from build123d import *

# Parameters (mm, degrees)
SKETCH1_W           = 56.388
SKETCH1_H           = 45.72
BOSS_EXTRUDE1_DEPTH = 2.54
SKETCH2_W           = 2.7432
SKETCH2_H           = 19.05
BOSS_EXTRUDE2_DEPTH = 2.54
SKETCH3_W           = 19.05
SKETCH3_H           = 2.7432
CUT_EXTRUDE1_DEPTH  = 3.54
SKETCH4_R           = 3.937
CUT_EXTRUDE2_DEPTH  = 3.54


with BuildPart() as part:
    # Sketch1 → Boss-Extrude1 (new body)
    with BuildSketch(Plane(origin=(0, 0, 0), x_dir=(0, 0, -1), z_dir=(1, 0, 0))):
        Rectangle(SKETCH1_W, SKETCH1_H)
    extrude(amount=BOSS_EXTRUDE1_DEPTH)

    # Sketch2 → Boss-Extrude2 (add)
    with BuildSketch(Plane(origin=(2.54, 0, 0), x_dir=(0, 0, -1), z_dir=(1, 0, 0))):
        with Locations((-29.5656, 0)):
            Rectangle(SKETCH2_W, SKETCH2_H)
        with Locations((29.5656, 0)):
            Rectangle(SKETCH2_W, SKETCH2_H)
    extrude(amount=-BOSS_EXTRUDE2_DEPTH)

    # Sketch3 → Cut-Extrude1 (cut, through all)
    with BuildSketch(Plane(origin=(2.54, 0, 0), x_dir=(0, 0, -1), z_dir=(1, 0, 0))):
        with Locations((0, 21.4884)):
            Rectangle(SKETCH3_W, SKETCH3_H)
        with Locations((0, -14.7066)):
            Rectangle(SKETCH3_W, SKETCH3_H)
    extrude(amount=-CUT_EXTRUDE1_DEPTH, mode=Mode.SUBTRACT)

    # Sketch4 → Cut-Extrude2 (cut, through all)
    with BuildSketch(Plane(origin=(2.54, 0, 0), x_dir=(0, 0, -1), z_dir=(1, 0, 0))):
        with Locations((11.8872, 10.16)):
            Circle(SKETCH4_R)
    extrude(amount=-CUT_EXTRUDE2_DEPTH, mode=Mode.SUBTRACT)


solid = part.part
Check sheet for the modelled part. Datum: model origin and axes. Units: mm. A direction names the side the tool comes from. Round coordinates to 2 decimals unless told otherwise and drop trailing zeros. Order: outer loops, then holes, each group sorted by start corner. A loop starts at its lowest first (then second) coordinate and runs counter-clockwise, first axis right, second up.
(1) Go/stop test with flat-tipped pins: P1, Ø1.3, axis at x = 2, y = -17.5, coming from the +Z side; P2, Ø0.8, axis at x = 1, z = 30, coming from the -Y side (3 decimals); P3, Ø1.3, axis at x = 0.5, z = 4, coming from the +Y side. Record where each tip stops, or that it passes through.
(2) Access from +Z, -Z, +X, -X, +Y, -Y to the whole of each face (thin tool, end or side, straight path). Record for faces 1 (the flat face through (1, 16, -28.194)), 2 (the flat face through (1, -16.078, 0)), 3 (the flat face through (1, -16, 28.194)), 4 (the flat face through (1, -16, -28.194)), 5 (the flat face through (1, 21, -9.525)).
(3) Cross-section at C-C, the plane x = 1.8. Enter the section's corners in (y, z) (3 decimals).
(4) Cross-section at A-A, the plane z = -2.5. Enter the section's corners in (x, y) (3 decimals).
(5) Scan lines: probe 1 along Y at (x, z) = (1.25, 6) (3 decimals); probe 2 along Z at (x, y) = (0.95, -13); probe 3 along Y at (x, z) = (1.6, -8.5) (3 decimals). Record each from-to range of solid material in increasing order.
(6) Cross-section at B-B, the plane y = 10.16. Enter the section's corners in (x, z).
(7) Draft check along Y on faces 6 (the flat face through (1, -15, 9.525)), 7 (the flat face through (1, 0, -30.937)), 8 (the flat face through (1, 20.117, 0)). Enter one of: pulls with the +Y half, pulls with the -Y half, needs draft (parallel to the pull), parting line crosses it, or undercut.
Check sheet entries:
1. P1: stops at z = 28.19
1. P2: stops at y = -9.525
1. P3: stops at y = 20.12
2. face 1: -Z, +X, -X, +Y
2. face 2: +X, -X
2. face 3: +Z, +X, -X, -Y
2. face 4: -Z, +X, -X, -Y
2. face 5: +X, -X, +Y
3. outline: (-22.86, -28.194) - (-9.525, -28.194) - (-9.525, -30.937) - (9.525, -30.937) - (9.525, -28.194) - (22.86, -28.194) - (22.86, -9.525) - (20.117, -9.525) - (20.117, 9.525) - (22.86, 9.525) - (22.86, 28.194) - (9.525, 28.194) - (9.525, 30.937) - (-9.525, 30.937) - (-9.525, 28.194) - (-22.86, 28.194) - close; hole (-16.078, -9.525) - (-13.335, -9.525) - (-13.335, 9.525) - (-16.078, 9.525) - close; hole circle Ø7.874 at (10.16, -11.887)
4. outline: (0, -22.86) - (2.54, -22.86) - (2.54, -16.078) - (0, -16.078) - close; (0, -13.335) - (2.54, -13.335) - (2.54, 20.117) - (0, 20.117) - close
5. probe 1: y = -22.86 to -16.078, -13.335 to 20.117
5. probe 2: z = -28.19 to 28.19
5. probe 3: y = -22.86 to -16.078, -13.335 to 8.153, 12.167 to 20.117
6. outline: (0, -28.19) - (2.54, -28.19) - (2.54, -15.82) - (0, -15.82) - close; (0, -7.95) - (2.54, -7.95) - (2.54, 28.19) - (0, 28.19) - close
7. face 6: undercut
7. face 7: needs draft
7. face 8: pulls with the +Y half
